Could you check a few things on this model? Use its own coordinates, in mm. A direction names the side the tool comes from. Give positions to 0.01 mm unless a question says otherwise; leave off trailing zeros. Order: outer loops, then holes, each group sorted by start corner. A loop starts at its lowest first (then second) coordinate and runs counter-clockwise, first axis right, second up.
from build123d import *

# Parameters (mm, degrees)
PAD_DEPTH         = 20
POCKET_DEPTH      = 6.001
POCKET_DEPTH_BACK = -31.001


with BuildPart() as part:
    # AdditivePipe: sweep along a path in Sketch
    with BuildLine(Plane.XY) as additivepipe_path:
        Line((0, 0), (0, 47))
    # Sketch001 → AdditivePipe (sweep)
    with BuildSketch(Plane.XZ):
        Polygon((-20, 6), (-20, -6), (-16, -6), (-9, -6), (9, -6), (16, -6), (20, -6), (20, 6), (16, 6), (16, 3), (9, 3), (-9, 3), (-16, 3), (-16, 6), align=None)
    sweep(path=additivepipe_path.line)

    # Sketch002 → Pad (new body, symmetric)
    with BuildSketch(Plane.YZ):
        Polygon((47, 6), (47, 17), (34, 31), (22, 31), (22, 17), (29, 17), (29, 3), (47, 3), align=None)
    extrude(amount=PAD_DEPTH, both=True)

    # Sketch003 → Pocket (cut, two sides)
    with BuildSketch(Plane.XY) as pocket_sk:
        with BuildLine():
            ThreePointArc((7, 12.362), (0, 19.362), (-7, 12.362))
            Line((-7, 12.362), (-7, 0))
            Line((-7, 0), (7, 0))
            Line((7, 12.362), (7, 0))
        make_face()
    extrude(amount=-POCKET_DEPTH, mode=Mode.SUBTRACT)
    extrude(pocket_sk.sketch, amount=-POCKET_DEPTH_BACK, mode=Mode.SUBTRACT)


solid = part.part
Item 1: Imagine slicing it at C-C on z = -2. List the corners of the cut face in (x, y) for me.
Findings:
outline: (-20, 0) - (-7, 0) - (-7, 12.36) arc R7 cw to (7, 12.36) - (7, 0) - (20, 0) - (20, 47) - (-20, 47) - close
Item 2: Imagine slicing it at D-D on y = 25.5. List the corners of the cut face in (x, z) for me, then the cut area to 3 significant figures.
Findings:
outline: (-20, -6) - (20, -6) - (20, 6) - (16, 6) - (16, 3) - (-16, 3) - (-16, 6) - (-20, 6) - close; (-20, 17) - (20, 17) - (20, 31) - (-20, 31) - close
area: 944 mm2
Item 3: Imagine slicing it at B-B on x = 0. List the corners of the cut face in (y, z) for me.
Findings:
outline: (19.36, -6) - (47, -6) - (47, 17) - (34, 31) - (22, 31) - (22, 17) - (29, 17) - (29, 3) - (19.36, 3) - close
Item 4: For faces 1 (the flat face through (-7, 6, -2)), 2 (the flat face through (-16, 15, 4)), 3 (the flat face through (0, 25, 17)), 4 (the flat face through (0, 22, 24)), which set-ups out of +Z, -Z, +X, -X, +Y, -Y let a thin tool reach every point of the face, with its end or its side?
Findings:
face 1: +Z, -Z, -Y
face 2: -Y
face 3: +X, -X, -Y
face 4: +Z, +X, -X, -Y
Item 5: Please list where these lines run through material, in increasing order: line 1 along Z through (x, y) = (-17.5, 25.5); line 2 along X through (y, z) = (8, -1.5); line 3 along Z through (x, y) = (8, 27.5).
Findings:
line 1: z = -6 to 6, 17 to 31
line 2: x = -20 to -7, 7 to 20
line 3: z = -6 to 3, 17 to 31
Item 6: We'd pull the mould along Z, two halves only. Please class faces 5 (the flat face through (18, 15, 6)), 6 (the flat face through (0, 21, 3)), 7 (the flat face through (0.28, 40.591, 23.902)), 8 (the cylindrical face through (0.15, 19.36, -1.44)): +Z half, -Z half, draft (parallel to the pull), parting line (faces both ways), or undercut.
Findings:
face 5: undercut
face 6: undercut
face 7: +Z half
face 8: draft
Item 7: Imagine slicing it at A-A on y = 3.5. List the corners of the cut face in (x, z) for me, then the cut area to 3 significant figures.
Findings:
outline: (-20, -6) - (-7, -6) - (-7, 3) - (-16, 3) - (-16, 6) - (-20, 6) - close; (7, -6) - (20, -6) - (20, 6) - (16, 6) - (16, 3) - (7, 3) - close
area: 258 mm2
Item 8: For pin 1 (6 mm diameter, centred on x = -1.5, z = 18.5, fed in from -Y); pin 2 (3 mm diameter, centred on x = -17, y = 19.5, fed in from +Z); pin 3 (11 mm diameter, centred on x = -6.5, z = 9, fed in from -Y); pin 4 (5 mm diameter, centred on x = 6, z = 0, fed in from -Y), each with a flat end and sliding along its axis, tell me the tip position at first contact or that it passes through.
Findings:
pin 1: stops at y = 22
pin 2: stops at z = 6
pin 3: stops at y = 29
pin 4: stops at y = 0
